Can you work these out from the drawing? Everything is in mm from the part's minimum corner. A direction names the side the tool comes from. Coordinates: 2 decimals unless noted, no trailing zeros. Write each loop counter-clockwise with the first axis right and the second up, starting at its lowest first coordinate (ties: lowest second). Pieces come first, ordered by that corner, then holes. Notation, with made-up numbers: M 33.25,-14.5 L 57.25,-14.5 A14 ccw 57.25,4.5 Z; hole C 55.5,41 d11. An arc over 180 degrees is marked long. Write item = value, one per line.
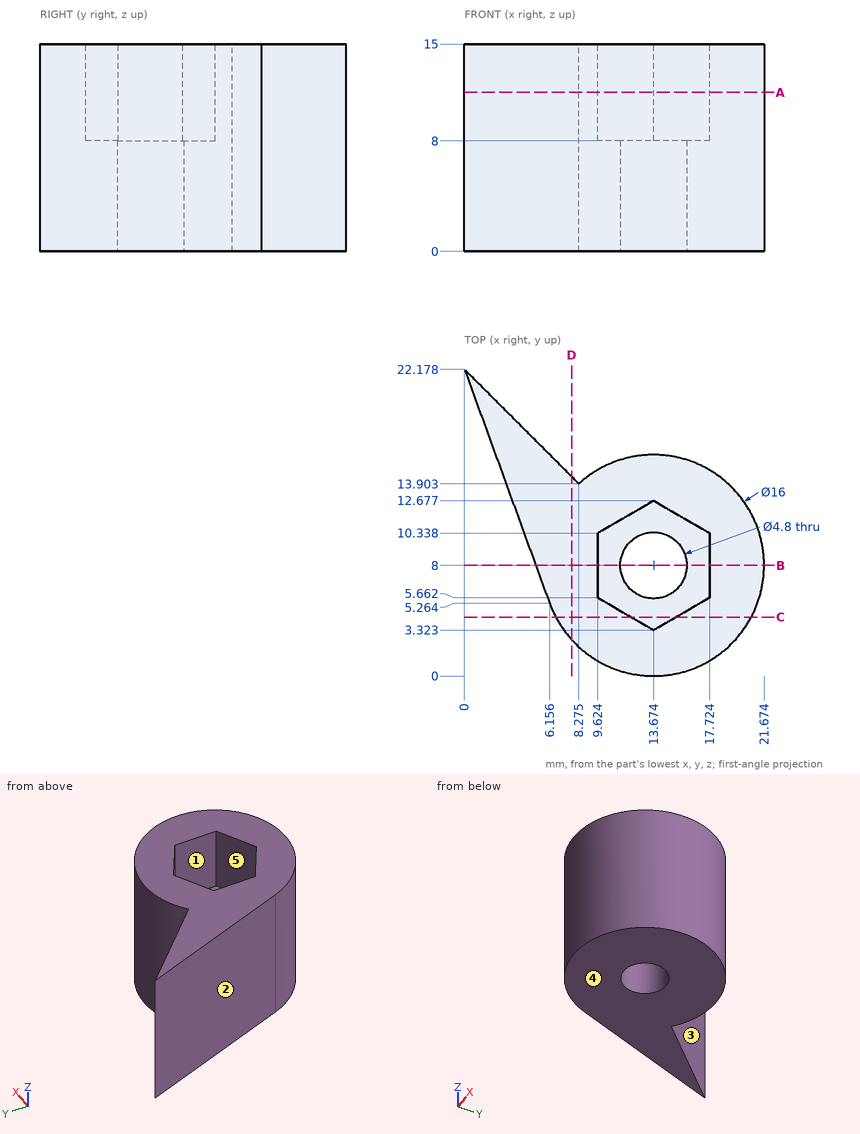
Item 1: Imagine slicing it at D-D (x = 7.75). Write out the boundary of the cut face in (y, z).
Numbers:
outline = M 2.62,0 L 14.43,0 L 14.43,15 L 2.62,15 Z
Item 2: I'm going to push flat-ended pins straight in: P1, Ø1.4, axis at y = 8, z = 11, coming from the -X side (1 decimal); P2, Ø6, axis at x = 10, z = 3.5, coming from the -Y side; P3, Ø1.5, axis at y = 3.5, z = 7, coming from the -X side; P4, Ø4, axis at y = 9, z = 7, coming from the +X side. Where does each tip first touch, or does it pass through?
Numbers:
P1 = 4.9
P2 = 0.03
P3 = 6.61
P4 = 21.67
Item 3: Imagine slicing it at B-B (y = 8). Write out the boundary of the cut face in (x, z), and give its area (3 significant figures).
Numbers:
outline = M 5.16,0 L 11.27,0 L 11.27,8 L 9.62,8 L 9.62,15 L 5.16,15 Z; M 16.07,0 L 21.67,0 L 21.67,15 L 17.72,15 L 17.72,8 L 16.07,8 Z
area = 153 mm²
Item 4: For the marked faces 1 and 2, which set-ups out of +Z, -Z, +X, -X, +Y, -Y let a thin tool reach every point of the face, with its end or its side?
Numbers:
face_1 = +Z
face_2 = +Z, -Z, -X, -Y
Item 5: If I drill on line 1 along Y through (x, z) = (13.5, 10.75) (1 decimal); line 2 along X through (y, z) = (7.75, 4); line 3 along Y through (x, z) = (17, 9.75) (1 decimal), over which ranges is the centre line in solid material (lowest first)?
Numbers:
line_1 = 0 to 3.4, 12.6 to 16
line_2 = 5.25 to 11.29, 16.06 to 21.67
line_3 = 0.7 to 5.2, 10.8 to 15.3
Item 6: Imagine slicing it at A-A (z = 11.5). Write out the boundary of the cut face in (x, y) (1 decimal).
Numbers:
outline = M 0,22.2 L 6.2,5.3 A8 ccw long 8.3,13.9 Z; hole M 9.6,5.7 L 13.7,3.3 L 17.7,5.7 L 17.7,10.3 L 13.7,12.7 L 9.6,10.3 Z
Item 7: If we mould it in two halves opening along Y, with no side actions, what happens to the marked faces 3, 4 and 5? For each: pulls with the +Y half, pulls with the -Y half, needs draft (parallel to the pull), parting line crosses it, or undercut.
Numbers:
face_3 = pulls with the +Y half
face_4 = needs draft
face_5 = undercut
Item 8: Imagine slicing it at C-C (y = 4.25). Write out the boundary of the cut face in (x, z).
Numbers:
outline = M 6.61,0 L 20.74,0 L 20.74,15 L 15.28,15 L 15.28,8 L 12.07,8 L 12.07,15 L 6.61,15 Z
